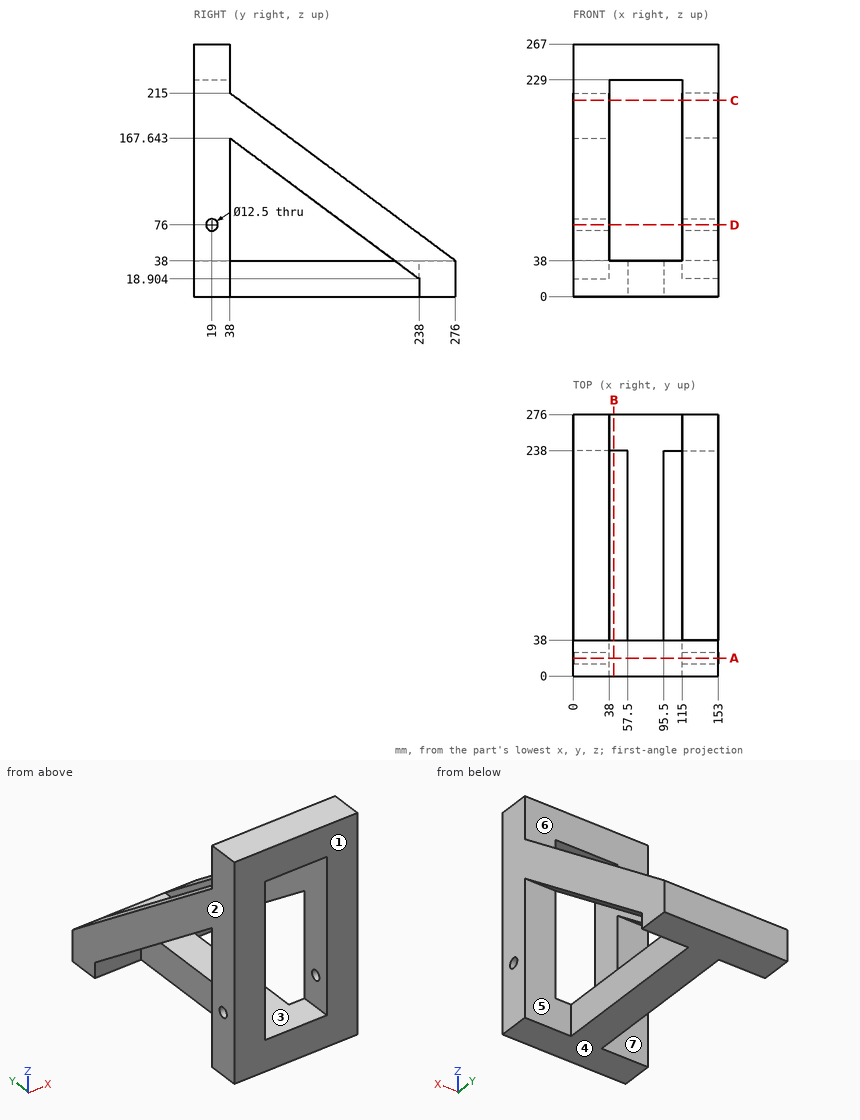
The drawing under review shows one solid part. Ordinate dimensions are in mm from its lowest x, y, z. A direction names the side the tool comes from. Round coordinates to 2 decimals unless told otherwise and drop trailing zeros. Loops run counter-clockwise (first coordinate to the right, second up) from the corner with the lowest first, then second, coordinate; pieces in that order, holes last.
Item 1: Mouldability with a two-part tool opening along X and no side actions: class the marked faces 1, 2 and 3 as released by +X, released by -X, zero draft, split by the parting line, or undercut.
Determined:
face 1: zero draft
face 2: released by -X
face 3: undercut
Item 2: Take a section at B-B (x = 43). Write out the cut boundary in (y, z).
Determined:
outline: (0, 0) - (38, 0) - (38, 38) - (0, 38) - close; (0, 229) - (38, 229) - (38, 267) - (0, 267) - close; (238, 0) - (276, 0) - (276, 38) - (238, 38) - close
Item 3: Take a section at A-A (y = 19). Write out the cut boundary in (x, z), then the cut area to 3 significant figures.
Determined:
outline: (0, 0) - (153, 0) - (153, 69.75) - (115, 69.75) - (115, 38) - (38, 38) - (38, 69.75) - (0, 69.75) - close; (0, 82.25) - (38, 82.25) - (38, 229) - (115, 229) - (115, 82.25) - (153, 82.25) - (153, 267) - (0, 267) - close
area: 25,200 mm2
Item 4: Take a section at D-D (z = 76). Write out the cut boundary in (x, y).
Determined:
outline: (0, 0) - (38, 0) - (38, 12.75) - (0, 12.75) - close; (0, 25.25) - (38, 25.25) - (38, 38) - (0, 38) - close; (0, 161.23) - (38, 161.23) - (38, 224.9) - (0, 224.9) - close; (115, 0) - (153, 0) - (153, 12.75) - (115, 12.75) - close; (115, 25.25) - (153, 25.25) - (153, 38) - (115, 38) - close; (115, 161.23) - (153, 161.23) - (153, 224.9) - (115, 224.9) - close
Item 5: Take a section at C-C (z = 207.5). Write out the cut boundary in (x, y) (1 decimal), then the cut area to 3 significant figures.
Determined:
outline: (0, 0) - (38, 0) - (38, 48.1) - (0, 48.1) - close; (115, 0) - (153, 0) - (153, 48.1) - (115, 48.1) - close
area: 3,650 mm2
Item 6: Clearance check with flat-ended pins moving along their axes: pin 1 Ø1 at (x, y) = (117.5, 175.5) entering from +Z; pin 2 Ø11.5 at (y, z) = (132, 22) entering from +X; pin 3 Ø19 at (y, z) = (101.5, 25.5) entering from -X; pin 4 Ø10 at (y, z) = (19, 76) entering from -X. State where each tip first meets the part, or that it passes through.
Determined:
pin 1: stops at z = 113.11
pin 2: stops at x = 95.5
pin 3: stops at x = 57.5
pin 4: passes through
Item 7: For the marked faces 4, 5, 6 and 7, list the 3-axis set-ups (+Z, -Z, +X, -X, +Y, -Y) from which the entire face can be reached by the end or side of a thin tool; tool diameter is ignored.
Determined:
face 4: -Z, +X, -X, +Y, -Y
face 5: -Z, +X
face 6: +Z, +X, -X, +Y
face 7: -Z, -X
Item 8: For line 1 (X direction, y = 71, z = 149); line 2 (Z direction, x = 75.5, y = 53.5), list the stretches that pass through material, from the lowest coordinate up.
Determined:
line 1: x = 0 to 38, 115 to 153
line 2: z = 0 to 38
